CAD build for the part. Positions are in the model's coordinates, mm. Face numbers are marked on the shaded views. A direction names the side the tool comes from. Round coordinates to 2 decimals unless told otherwise and drop trailing zeros. Order: outer loops, then holes, each group sorted by start corner. A loop starts at its lowest first (then second) coordinate and runs counter-clockwise, first axis right, second up. Notation, with made-up numbers: M 78.5,-31.75 L 137.5,-31.75 A34 cw 137.5,1.25 Z; hole C -24.5,13.5 d8. An arc over 180 degrees is marked long. Put each result on its own line as item: value.
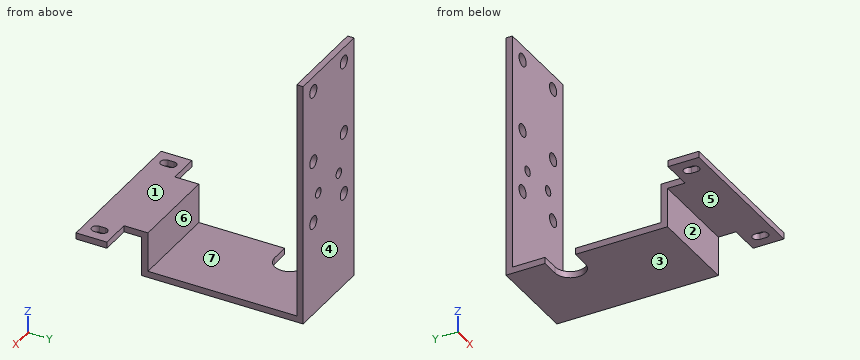
```python
from build123d import *

# Parameters (mm, degrees)
F0_W      = 30
F0_H      = 81
F1_DEPTH  = 2.1
F2_W      = 30
F2_H      = 2.1
F3_DEPTH  = 51.2
F4_W      = 30
F4_H      = 2.1
F5_DEPTH  = 13.1
F6_W      = 30
F6_H      = 2.1
F7_DEPTH  = 16
F8_W      = 10.1
F8_H      = 10.2
F9_DEPTH  = 2.1
F11_DEPTH = 15.201
F13_DEPTH = 2.101
F14_R     = 2.1
F14_R_2   = 1.6
F15_DEPTH = 2.101


with BuildPart() as f1:
    # F0 (on Front) → F1 (new body)
    with BuildSketch(Plane.XZ):
        Rectangle(F0_W, F0_H)
    extrude(amount=F1_DEPTH)

    # F2 (on face) → F3 (join)
    with BuildSketch(Plane.XZ.offset(2.1)):
        with Locations((0, -39.45)):
            Rectangle(F2_W, F2_H)
    extrude(amount=F3_DEPTH)

    # F4 (on face) → F5 (join)
    with BuildSketch(Plane.XY.offset(-38.4)):
        with Locations((0, -52.25)):
            Rectangle(F4_W, F4_H)
    extrude(amount=F5_DEPTH)

    # F6 (on face) → F7 (join)
    with BuildSketch(Plane.XZ.offset(53.3)):
        with Locations((0, -26.35)):
            Rectangle(F6_W, F6_H)
    extrude(amount=F7_DEPTH)

    # F8 (on face) → F9 (join)
    with BuildSketch(Plane.XY.offset(-25.3)):
        with Locations((-20.05, -64.2)):
            Rectangle(F8_W, F8_H)
        with Locations((20.05, -64.2)):
            Rectangle(F8_W, F8_H)
    extrude(amount=-F9_DEPTH)

    # F10 (on face) → F11 (cut, through all)
    with BuildSketch(Plane.XY.offset(-25.3)):
        with BuildLine():
            Line((-21.9, -63.2), (-21.9, -65.2))
            ThreePointArc((-21.9, -65.2), (-20.3, -66.8), (-18.7, -65.2))
            Line((-18.7, -65.2), (-18.7, -63.2))
            ThreePointArc((-18.7, -63.2), (-20.3, -61.6), (-21.9, -63.2))
        make_face()
        with BuildLine():
            Line((18.7, -63.2), (18.7, -65.2))
            ThreePointArc((18.7, -65.2), (20.3, -66.8), (21.9, -65.2))
            Line((21.9, -65.2), (21.9, -63.2))
            ThreePointArc((21.9, -63.2), (20.3, -61.6), (18.7, -63.2))
        make_face()
    extrude(amount=-F11_DEPTH, mode=Mode.SUBTRACT)

    # F12 (on face) → F13 (cut, through all)
    with BuildSketch(Plane.XY.offset(-38.4)):
        with BuildLine():
            Line((-15, -22.894339), (-9.15, -22.894339))
            ThreePointArc((-9.15, -22.894339), (-4.15, -17.894339), (-9.15, -12.894339))
            Line((-9.15, -12.894339), (-15, -12.894339))
            Line((-15, -12.894339), (-15, -22.894339))
        make_face()
    extrude(amount=-F13_DEPTH, mode=Mode.SUBTRACT)

    # F14 (on face) → F15 (cut, through all)
    with BuildSketch(Plane.XZ.offset(2.1)):
        with Locations((9, 35.6)):
            Circle(F14_R)
        with Locations((9, 11.6)):
            Circle(F14_R)
        with Locations((-9, 35.6)):
            Circle(F14_R)
        with Locations((-9, 11.6)):
            Circle(F14_R)
        with Locations((9, -9.2)):
            Circle(F14_R)
        with Locations((-9, -9.2)):
            Circle(F14_R)
        with Locations((6.05, -0.7)):
            Circle(F14_R_2)
        with Locations((-6.05, -0.7)):
            Circle(F14_R_2)
    extrude(amount=-F15_DEPTH, mode=Mode.SUBTRACT)


solid = f1.part
```
Item 1: Band-saw the part on B-B on x = 9. Give the cut face in (y, z).
Answers below:
outline: M -69.3,-27.4 L -53.3,-27.4 L -53.3,-40.5 L 0,-40.5 L 0,-11.3 L -2.1,-11.3 L -2.1,-38.4 L -51.2,-38.4 L -51.2,-25.3 L -69.3,-25.3 Z; M -2.1,-7.1 L 0,-7.1 L 0,9.5 L -2.1,9.5 Z; M -2.1,13.7 L 0,13.7 L 0,33.5 L -2.1,33.5 Z; M -2.1,37.7 L 0,37.7 L 0,40.5 L -2.1,40.5 Z
Item 2: Mould opens along Y. For the marked faces 4, 5, 6 and 7 say: pulls with the +Y half, pulls with the -Y half, needs draft (parallel to the pull), parting line crosses it, or undercut.
Answers below:
face 4: pulls with the +Y half
face 5: needs draft
face 6: undercut
face 7: undercut
Item 3: Pin check, flat tips, straight feed: P1, Ø6.5, axis at x = -9, z = -9.2, coming from the -Y side; P2, Ø13, axis at x = 4, y = -64.5, coming from the -Z side; P3, Ø4, axis at x = 9, z = -9.2, coming from the +Y side; P4, Ø1.5, axis at x = -4, y = -61.5, coming from the +Z side. Stop position of each tip, or through.
Answers below:
P1: y = -2.1
P2: z = -27.4
P3: through
P4: z = -25.3
Item 4: Tool access for the marked faces 1, 2 and 3: list every direction of +Z, -Z, +X, -X, +Y, -Y with a clear straight run to the whole face (end or side of a thin tool).
Answers below:
face 1: +Z, +X, -X, -Y
face 2: -Z, +X, -X, -Y
face 3: -Z, +X, -X, +Y, -Y
Item 5: Band-saw the part on A-A on z = -32. Give the cut face in (x, y), and give its area (3 significant figures).
Answers below:
outline: M -15,-53.3 L 15,-53.3 L 15,-51.2 L -15,-51.2 Z; M -15,-2.1 L 15,-2.1 L 15,0 L -15,0 Z
area: 126 mm²
Item 6: Probe line 1 along Z through (x, y) = (-9, -1.1); line 2 along Y through (x, z) = (-9, -34.5); line 3 along Z through (x, y) = (-6.05, -0.8). List the from-to ranges inside material, lowest first. Write a range as [from, to].
Answers below:
line 1: [-40.5, -11.3], [-7.1, 9.5], [13.7, 33.5], [37.7, 40.5]
line 2: [-53.3, -51.2], [-2.1, 0]
line 3: [-40.5, -2.3], [0.9, 40.5]
Item 7: Band-saw the part on C-C on z = -0.7. Give the cut face in (x, y).
Answers below:
outline: M -15,-2.1 L -7.65,-2.1 L -7.65,0 L -15,0 Z; M -4.45,-2.1 L 4.45,-2.1 L 4.45,0 L -4.45,0 Z; M 7.65,-2.1 L 15,-2.1 L 15,0 L 7.65,0 Z
Item 8: Band-saw the part on D-D on x = -12.5. Give the cut face in (y, z), and give its area (3 significant figures).
Answers below:
outline: M -69.3,-27.4 L -53.3,-27.4 L -53.3,-40.5 L -22.89,-40.5 L -22.89,-38.4 L -51.2,-38.4 L -51.2,-25.3 L -69.3,-25.3 Z; M -12.89,-40.5 L 0,-40.5 L 0,40.5 L -2.1,40.5 L -2.1,-38.4 L -12.89,-38.4 Z
area: 318 mm²
